Model file for the job. Use its own axes, mm. Face numbers are marked on the shaded views. A direction names the side the tool comes from. Give positions to 0.01 mm unless a question says otherwise; leave off trailing zeros. Write each loop counter-clockwise with the first axis right and the second up, starting at its lowest first coordinate (ties: lowest second). Pieces come first, ordered by that corner, then holes.
```python
from build123d import *

# Parameters (mm, degrees)
SKIZZE1_W                       = 18
SKIZZE1_H                       = 11
SKIZZE1_R                       = 2.2
AUFSATZ_LINEAR_AUSTRAGEN1_DEPTH = 7.5
SKIZZE2_R                       = 4.5
SCHNITT_LINEAR_AUSTRAGEN1_DEPTH = 3.5


with BuildPart() as part:
    # Skizze1 → Aufsatz-Linear austragen1 (new body)
    with BuildSketch(Plane.XY):
        Rectangle(SKIZZE1_W, SKIZZE1_H)
        Circle(SKIZZE1_R, mode=Mode.SUBTRACT)
    extrude(amount=AUFSATZ_LINEAR_AUSTRAGEN1_DEPTH)

    # Skizze2 → Schnitt-Linear austragen1 (cut)
    with BuildSketch(Plane.XY.offset(7.5)):
        Circle(SKIZZE2_R)
    extrude(amount=-SCHNITT_LINEAR_AUSTRAGEN1_DEPTH, mode=Mode.SUBTRACT)

    # Spiegeln1: part across plane


with BuildPart() as part_1:
    add(part.part)
    add(part.part.mirror(Plane(origin=(-9, -5.5, 7.5), x_dir=(0, 0, 1), z_dir=(0, 1, 0))))


solid = part_1.part
```
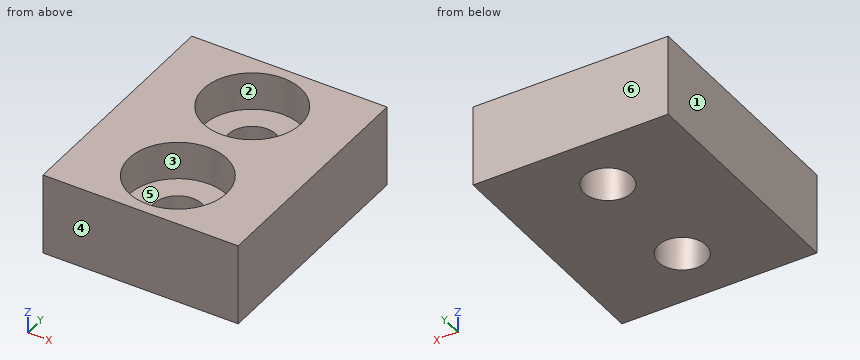
1. Slice it at B-B, the plane x = 0. Write the cut outline in (y, z).
Calculated:
outline: (-16.5, 0) - (-13.2, 0) - (-13.2, 4) - (-15.5, 4) - (-15.5, 7.5) - (-16.5, 7.5) - close; (-8.8, 0) - (-2.2, 0) - (-2.2, 4) - (-4.5, 4) - (-4.5, 7.5) - (-6.5, 7.5) - (-6.5, 4) - (-8.8, 4) - close; (2.2, 0) - (5.5, 0) - (5.5, 7.5) - (4.5, 7.5) - (4.5, 4) - (2.2, 4) - close
2. Slice it at D-D, the plane x = 3. Write the cut outline in (y, z).
Calculated:
outline: (-16.5, 0) - (5.5, 0) - (5.5, 7.5) - (3.35, 7.5) - (3.35, 4) - (-3.35, 4) - (-3.35, 7.5) - (-7.65, 7.5) - (-7.65, 4) - (-14.35, 4) - (-14.35, 7.5) - (-16.5, 7.5) - close
3. Pin check, flat tips, straight feed: P1, Ø7, axis at x = 0, y = 0, coming from the -Z side; P2, Ø4.5, axis at x = -1, y = 0, coming from the +Z side. Stop position of each tip, or through.
Calculated:
P1: stops at z = 0
P2: stops at z = 4
4. Slice it at C-C, the plane z = 3.25. Write the cut outline in (x, y), and give its area (3 significant figures).
Calculated:
outline: (-9, -16.5) - (9, -16.5) - (9, 5.5) - (-9, 5.5) - close; hole circle Ø4.4 at (0, -11); hole circle Ø4.4 at (0, 0)
area: 366 mm2
5. Probe probe 1 along Y at (x, z) = (0, 3.2); probe 2 along Y at (x, z) = (0, 6.3); probe 3 along X at (y, z) = (-11, 5.8). List the from-to ranges inside material, lowest first.
Calculated:
probe 1: y = -16.5 to -13.2, -8.8 to -2.2, 2.2 to 5.5
probe 2: y = -16.5 to -15.5, -6.5 to -4.5, 4.5 to 5.5
probe 3: x = -9 to -4.5, 4.5 to 9
6. Pull direction Y, two halves, no side cores. Call the marked faces 1, 2, 3 and 4: +Y half, -Y half, draft (parallel to the pull), parting line (faces both ways), or undercut.
Calculated:
face 1: draft
face 2: undercut
face 3: undercut
face 4: -Y half
7. Which spindle directions (+Z, -Z, +X, -X, +Y, -Y) get a long thin tool onto all of the face, cutting with end or side? Do the marked faces 5 and 6. Say none if no direction does.
Calculated:
face 5: +Z
face 6: +Z, -Z, +X, -X, +Y
8. Slice it at A-A, the plane y = 0. Write the cut outline in (x, z), and give its area (3 significant figures).
Calculated:
outline: (-9, 0) - (-2.2, 0) - (-2.2, 4) - (-4.5, 4) - (-4.5, 7.5) - (-9, 7.5) - close; (2.2, 0) - (9, 0) - (9, 7.5) - (4.5, 7.5) - (4.5, 4) - (2.2, 4) - close
area: 85.9 mm2
